Design review of the part built by this model. Coordinates are the model's own, in mm. A direction names the side the tool comes from. Give positions to 0.01 mm unless a question says otherwise; leave off trailing zeros. Write each loop counter-clockwise with the first axis right and the second up, starting at its lowest first coordinate (ties: lowest second). Pieces come first, ordered by that corner, then holes. Notation, with made-up numbers: M 17,57 L 39,57 A31 cw 39,93 Z; hole C 13.25,36.25 d9. An arc over 180 degrees is marked long. Use a Markdown table: item, result. Add a question column.
```python
from build123d import *

# Parameters (mm, degrees)
F0_R     = 2
F1_DEPTH = 5.57


with BuildPart() as f1:
    # F0 (on Top) → F1 (new body)
    with BuildSketch(Plane.XY):
        with BuildLine():
            ThreePointArc((-11.400436, 18.726019), (-9.907034, 20.19309), (-9.359215, 22.213595))
            ThreePointArc((-9.359215, 22.213595), (-10.128315, 24.571832), (-12.139857, 26.02321))
            ThreePointArc((-12.139857, 26.02321), (-14.752933, 25.962935), (-16.770909, 24.301739))
            ThreePointArc((-16.770909, 24.301739), (-17.330326, 21.73372), (-16.175298, 19.372877))
            ThreePointArc((-16.175298, 19.372877), (-13.896196, 18.249802), (-11.400436, 18.726019))
        make_face()
        with Locations((-13.359215, 22.213595)):
            Circle(F0_R, mode=Mode.SUBTRACT)
        with BuildLine():
            ThreePointArc((-16.770909, 24.301739), (-14.752933, 25.962935), (-12.139857, 26.02321))
            Line((-12.139857, 26.02321), (-12.139857, 37.861944))
            Line((-12.139857, 37.861944), (-16.770909, 30.644984))
            Line((-16.770909, 30.644984), (-16.770909, 24.301739))
        make_face()
        with BuildLine():
            add(Edge.make_bspline(
                [(-11.400436, 18.726019), (-10.838788, 14.530542), (-5.788488, 8.946827), (0, 2.861944)],
                knots=[0, 0, 0, 0, 19.535578, 19.535578, 19.535578, 19.535578], degree=3))
            ThreePointArc((-11.400436, 18.726019), (-13.896196, 18.249802), (-16.175298, 19.372877))
            add(Edge.make_bspline(
                [(-16.175298, 19.372877), (-15.218746, 9.630905), (-9.362263, 8.004596), (0, 2.861944)],
                knots=[0, 0, 0, 0, 23.113874, 23.113874, 23.113874, 23.113874], degree=3))
        make_face()
    extrude(amount=F1_DEPTH)


solid = f1.part
```
(1) Add section A-A on y = 23. Give the boundary of the cut face in (x, z).
(2) The part is to be moulded in two halves that separate along Y. For faces 3 (the cylindrical face through (-11.51, 21.45, 2.75)), 4 (the flat face through (-14.423, 34.304, 2.746)), 5 (the flat face through (-16.771, 28, 3)), 6 (the cylindrical face through (-17.335, 21.771, 2.746)), say which applies: released by +Y, released by -Y, zero draft, split by the parting line, or undercut.
(3) Wall thickness on L1, parallel to X at y = 24, z = 4.75; L2, parallel to X at y = 21, z = 2.5; L3, parallel to Y at x = -14.25, z = 1.25: over which ranges is each line inside the solid? List them lowest first.
(4) For pin 1 (1.5 mm diameter, centred on y = 8.5, z = 1.5, fed in from -X); pin 2 (1 mm diameter, centred on y = 30, z = 2, fed in from +X); pin 3 (1 mm diameter, centred on y = 20, z = 1, fed in from -X), all flat-tipped, find the tip position at first contact; note any pin that passes through.
(5) Add section B-B on y = 30. Give the boundary of the cut face in (x, z), then the cut area to 3 significant figures.
(6) Machinability: for faces 1 (the flat face through (-12.14, 32, 3)), 2 (the flat face through (-12, 19, 5.57)), which of the approach directions +Z, -Z, +X, -X, +Y, -Y give a long, thin tool a straight path to every point of the face, cutting with its end or side? Answer none if there is none.
From the geometry:
| question | item | result |
|---|---|---|
| 1 | outline | M -17.28,0 L -15.2,0 L -15.2,5.57 L -17.28,5.57 Z; M -11.52,0 L -9.44,0 L -9.44,5.57 L -11.52,5.57 Z |
| 2 | face 3 | undercut |
| 2 | face 4 | released by +Y |
| 2 | face 5 | zero draft |
| 2 | face 6 | split by the parting line |
| 3 | L1 | x = -16.94 to -14.26, -12.46 to -9.78 |
| 3 | L2 | x = -17.17 to -14.95, -11.77 to -9.55 |
| 3 | L3 | y = 12.84 to 20.42, 24 to 34.57 |
| 4 | pin 1 | stops at x = -11.06 |
| 4 | pin 2 | stops at x = -12.14 |
| 4 | pin 3 | stops at x = -16.97 |
| 5 | outline | M -16.77,0 L -12.14,0 L -12.14,5.57 L -16.77,5.57 Z |
| 5 | area | 25.8 mm^2 |
| 6 | face 1 | +Z, -Z, +X, +Y |
| 6 | face 2 | +Z, +X, -X, +Y, -Y |
